Geometry check sheet. Reference: the model listing, model coordinates, mm. A direction names the side the tool comes from. Round coordinates to 2 decimals unless told otherwise and drop trailing zeros. Write each loop counter-clockwise with the first axis right and the second up, starting at its lowest first coordinate (ties: lowest second). Pieces come first, ordered by that corner, then holes. Notation, with made-up numbers: (-33, 4) - (-29, 4) arc R21 cw to (-29, 40) - close; hole circle Ø5 at (50.25, 41). An arc over 180 degrees is marked (long way). Return JSON: item names as keys, results as strings.
```python
from build123d import *

# Parameters (mm, degrees)
F0_R     = 2.5
F1_DEPTH = 3


with BuildPart() as f1:
    # F0 (on Right) → F1 (new body)
    with BuildSketch(Plane.YZ):
        Polygon((30, -14), (30, 21), (15, 21), (15, 18), (-65, 18), (-65, 21), (-80, 21), (-80, -79), (-65, -79), (-65, -76), (15, -76), (15, -79), (30, -79), (30, -44), (33, -44), (33, -14), align=None)
        with Locations((-73, 0)):
            Circle(F0_R, mode=Mode.SUBTRACT)
        with Locations((-63, 0)):
            Circle(F0_R, mode=Mode.SUBTRACT)
        with Locations((-53, 0)):
            Circle(F0_R, mode=Mode.SUBTRACT)
        with BuildLine():
            Line((0, 4.025), (20, 4.025))
            ThreePointArc((20, 4.025), (24.025, 0), (20, -4.025))
            Line((20, -4.025), (0, -4.025))
            ThreePointArc((0, -4.025), (-4.025, 0), (0, 4.025))
        make_face(mode=Mode.SUBTRACT)
    extrude(amount=F1_DEPTH)


solid = f1.part
```
(1) Section check D-D, the plane y = -25. Enter the section's corners in (x, z), plus the area to 3 significant figures.
Response values:
{"outline": "(0, -76) - (3, -76) - (3, 18) - (0, 18) - close", "area": "282 mm^2"}
(2) Release check for a two-part mould opening along Y. For faces 5 (the face through (1.48, -60.69, -0.96)), 6 (the face through (1, 30, 3)), 7 (the face through (3, -24, -28)) record: pulls with the +Y half, pulls with the -Y half, needs draft (parallel to the pull), parting line crosses it, or undercut.
Response values:
{"face 5": "undercut", "face 6": "pulls with the +Y half", "face 7": "needs draft"}
(3) Access from +Z, -Z, +X, -X, +Y, -Y to the whole of each face (thin tool, end or side, straight path). Record for faces 1 (the face through (1, 32, -14)), 2 (the face through (1, -65, -78)), 3 (the face through (1, 15, 20)), 4 (the face through (1.479, -4.024, -0.089)).
Response values:
{"face 1": "+Z, +X, -X, +Y", "face 2": "-Z, +X, -X", "face 3": "+Z, +X, -X", "face 4": "+X, -X"}
(4) Material ranges on line 1 along Z through (x, y) = (2.1, -63); line 2 along Z through (x, y) = (1.7, 2.5) (3 decimals); line 3 along Y through (x, z) = (1.15, -59), recorded low to high. Write a range as [from, to].
Response values:
{"line 1": "z = [-76, -2.5], [2.5, 18]", "line 2": "z = [-76, -4.025], [4.025, 18]", "line 3": "y = [-80, 30]"}
(5) Section check B-B, the plane x = 1.3. Enter the section's corners in (y, z) (3 decimals).
Response values:
{"outline": "(-80, -79) - (-65, -79) - (-65, -76) - (15, -76) - (15, -79) - (30, -79) - (30, -44) - (33, -44) - (33, -14) - (30, -14) - (30, 21) - (15, 21) - (15, 18) - (-65, 18) - (-65, 21) - (-80, 21) - close; hole circle Ø5 at (-73, 0); hole circle Ø5 at (-63, 0); hole circle Ø5 at (-53, 0); hole (0, -4.025) - (20, -4.025) arc R4.025 ccw to (20, 4.025) - (0, 4.025) arc R4.025 ccw to start"}
(6) Gauge pin test, flat ends, axial feed: pin 1 (0.9 mm diameter, centred on x = 1.5, y = -22, fed in from -Z); pin 2 (6 mm diameter, centred on y = -53, z = 0, fed in from -X); pin 3 (0.9 mm diameter, centred on x = 1, z = 2, fed in from +Y); pin 4 (0.9 mm diameter, centred on x = 1.5, y = 10, fed in from +Z). Record the tip position at first contact, or that the pin passes through.
Response values:
{"pin 1": "stops at z = -76", "pin 2": "stops at x = 0", "pin 3": "stops at y = 30", "pin 4": "stops at z = 18"}
(7) Section check A-A, the plane z = 0. Enter the section's corners in (x, y) (3 decimals), plus the area to 3 significant figures.
Response values:
{"outline": "(0, -80) - (3, -80) - (3, -75.5) - (0, -75.5) - close; (0, -70.5) - (3, -70.5) - (3, -65.5) - (0, -65.5) - close; (0, -60.5) - (3, -60.5) - (3, -55.5) - (0, -55.5) - close; (0, -50.5) - (3, -50.5) - (3, -4.025) - (0, -4.025) - close; (0, 24.025) - (3, 24.025) - (3, 30) - (0, 30) - close", "area": "201 mm^2"}
(8) Section check C-C, the plane y = -53. Enter the section's corners in (x, z), plus the area to 3 significant figures.
Response values:
{"outline": "(0, -76) - (3, -76) - (3, -2.5) - (0, -2.5) - close; (0, 2.5) - (3, 2.5) - (3, 18) - (0, 18) - close", "area": "267 mm^2"}
